The model under review builds one solid part; all positions refer to its coordinate system, in mm. A direction names the side the tool comes from. Coordinates: 2 decimals unless noted, no trailing zeros. Write each loop counter-clockwise with the first axis right and the second up, starting at its lowest first coordinate (ties: lowest second). Pieces come first, ordered by that corner, then holes.
```python
from build123d import *

# Parameters (mm, degrees)
BOSS_EXTRUDE1_DEPTH = 25
SKETCH2_R           = 2.5
CUT_EXTRUDE1_DEPTH  = 90.489411687


with BuildPart() as part:
    # Sketch1 → Boss-Extrude1 (new body)
    with BuildSketch(Plane.XY):
        Polygon((0, 0), (55.236413043, 0), (55.236413043, 15), (81.236413043, 15), (81.236413043, 28), (41.236413043, 28), (25.236413043, 13), (-24.763586957, 13), (-24.763586957, 0), align=None)
    extrude(amount=BOSS_EXTRUDE1_DEPTH)

    # Sketch2 → Cut-Extrude1 (cut, through all)
    with BuildSketch(Plane(origin=(0, 28, 0), x_dir=(1, 0, 0), z_dir=(0, 1, 0))):
        with Locations(Location((76.236413043, -12.5, 0), (0, 0, 180))):
            Circle(SKETCH2_R)
        with Locations(Location((61.236413043, -12.5, 0), (0, 0, 180))):
            Circle(SKETCH2_R)
    extrude(amount=-CUT_EXTRUDE1_DEPTH, mode=Mode.SUBTRACT)


solid = part.part
```
Item 1: Take a section at B-B, the plane z = 5. Write out the cut boundary in (x, y).
Solved:
outline: (-24.76, 0) - (55.24, 0) - (55.24, 15) - (81.24, 15) - (81.24, 28) - (41.24, 28) - (25.24, 13) - (-24.76, 13) - close
Item 2: Machinability: for faces 4 (the face through (68, 15, 12)), 5 (the face through (1, 13, 12)), 6 (the face through (-24.764, 7, 12)), which of the approach directions +Z, -Z, +X, -X, +Y, -Y give a long, thin tool a straight path to every point of the face, cutting with its end or side? Answer none if there is none.
Solved:
face 4: +Z, -Z, +X, -Y
face 5: +Z, -Z, -X, +Y
face 6: +Z, -Z, -X, +Y, -Y
Item 3: Mouldability with a two-part tool opening along X and no side actions: class faces 1 (the face through (55.236, 7, 12)), 2 (the face through (58.93, 21.59, 11.54)), 3 (the face through (61.5, 28, 9.5)) as pulls with the +X half, pulls with the -X half, needs draft (parallel to the pull), parting line crosses it, or undercut.
Solved:
face 1: pulls with the +X half
face 2: undercut
face 3: needs draft
Item 4: Take a section at D-D, the plane x = 11.5. Write out the cut boundary in (y, z).
Solved:
outline: (0, 0) - (13, 0) - (13, 25) - (0, 25) - close
Item 5: Take a section at A-A, the plane z = 12.5. Write out the cut boundary in (x, y).
Solved:
outline: (-24.76, 0) - (55.24, 0) - (55.24, 15) - (58.74, 15) - (58.74, 28) - (41.24, 28) - (25.24, 13) - (-24.76, 13) - close; (63.74, 15) - (73.74, 15) - (73.74, 28) - (63.74, 28) - close; (78.74, 15) - (81.24, 15) - (81.24, 28) - (78.74, 28) - close
Item 6: For pin 1 (1.5 mm diameter, centred on x = 60, z = 4, fed in from -Y); pin 2 (1.5 mm diameter, centred on y = 4.5, z = 15, fed in from +X), all flat-tipped, find the tip position at first contact; note any pin that passes through.
Solved:
pin 1: stops at y = 15
pin 2: stops at x = 55.24
Item 7: Take a section at C-C, the plane y = 22.75. Write out the cut boundary in (x, z).
Solved:
outline: (35.64, 0) - (81.24, 0) - (81.24, 25) - (35.64, 25) - close; hole circle Ø5 at (61.24, 12.5); hole circle Ø5 at (76.24, 12.5)
Item 8: To check wall thickness, follow line 1 along X through (y, z) = (15.75, 10.25); line 2 along Y through (x, z) = (-15.5, 15); line 3 along Y through (x, z) = (68.5, 4.75). State the ranges of each line that lie inside material, in increasing order.
Solved:
line 1: x = 28.17 to 60.15, 62.33 to 75.15, 77.33 to 81.24
line 2: y = 0 to 13
line 3: y = 15 to 28
